Job drawing, mm, ordinate dimensions from the low corner. One solid piece. Coordinates: 2 decimals unless noted, no trailing zeros. Loops run counter-clockwise (first coordinate to the right, second up) from the corner with the lowest first, then second, coordinate; pieces in that order, holes last. Notation, with made-up numbers: (31, 55) -> (51, 55) arc R12 ccw to (51, 76) -> close; hole circle Ø7 at (7, 65.5). An arc over 180 degrees is marked (long way). Use one line per item in the form item = value. Start each with the question number.
(1) Band-saw the part on A-A on z = 12.5. Give the cut face in (x, y).
(2) Band-saw the part on D-D on x = 498. Give the cut face in (y, z), then the cut area to 3 significant figures.
(3) Band-saw the part on B-B on x = 210. Give the cut face in (y, z), then the cut area to 3 significant figures.
(4) Drill centre lines: L1, parallel to Y at x = 280, z = 14; L2, parallel to X at y = 281, z = 6.5; L3, parallel to Y at x = 280, z = 4. Where is each one in solid material? Low to high. Write a range as [from, to].
(5) Pin check, flat tips, straight feed: P1, Ø3, axis at x = 62.5, z = 9.5, coming from the -Y side; P2, Ø1, axis at y = 83, z = 7.5, coming from the +X side; P3, Ø2, axis at y = 200.5, z = 13.5, coming from the -X side. Stop position of each tip, or through.
(6) Band-saw the part on C-C on y = 348.5. Give the cut face in (x, z), then the cut area to 3 significant figures.
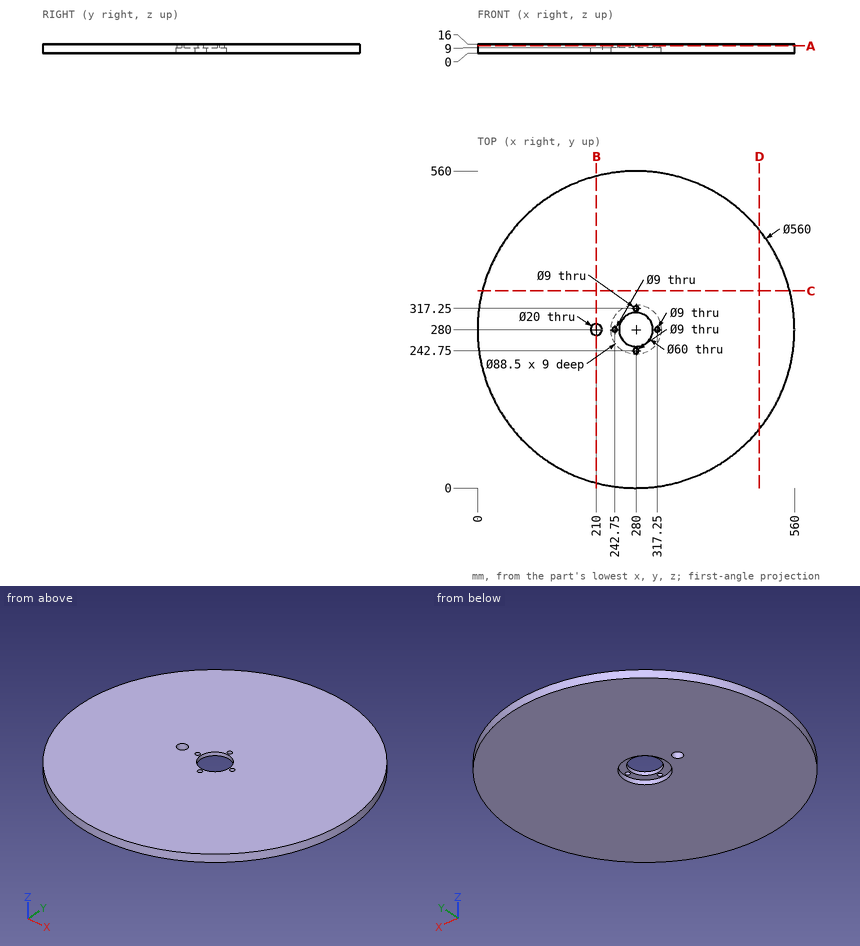
A:
q1.outline = circle Ø560 at (280, 280); hole circle Ø20 at (210, 280); hole circle Ø9 at (242.75, 280); hole circle Ø60 at (280, 280); hole circle Ø9 at (280, 242.75); hole circle Ø9 at (280, 317.25); hole circle Ø9 at (317.25, 280)
q2.outline = (104.28, 0) -> (455.72, 0) -> (455.72, 16) -> (104.28, 16) -> close
q2.area = 5,620 mm²
q3.outline = (8.89, 0) -> (270, 0) -> (270, 16) -> (8.89, 16) -> close; (290, 0) -> (551.11, 0) -> (551.11, 16) -> (290, 16) -> close
q3.area = 8,360 mm²
q4.L1 = [0, 238.25], [247.25, 250], [310, 312.75], [321.75, 560]
q4.L2 = [0, 200.05], [219.95, 235.76], [324.24, 560]
q4.L3 = [0, 235.75], [324.25, 560]
q5.P1 = 101.83
q5.P2 = 479.47
q5.P3 = 11.23
q6.outline = (8.51, 0) -> (551.49, 0) -> (551.49, 16) -> (8.51, 16) -> close
q6.area = 8,690 mm²
